Here's how the part is built. I have some questions about the finished solid (model axes, mm). A direction names the side the tool comes from. Give positions to 0.01 mm unless a question says otherwise; leave off trailing zeros. Write each loop counter-clockwise with the first axis right and the second up, starting at its lowest first coordinate (ties: lowest second). Pieces come first, ordered by that corner, then holes. Notation, with made-up numbers: (22.25, -35.75) - (38.25, -35.75) arc R19 cw to (38.25, -0.75) - close; hole circle Ø1 at (67, 33.5). An arc over 180 degrees is marked (long way). One line per item, written item: value. Start each with the question number.
1) On a 3-axis mill with a long thin cutter (end or side, diameter ignored), from which of +Z, -Z, +X, -X, +Y, -Y can I reach the whole of each face in a straight line? I mean faces 1 (the cylindrical face through (20.047, 1.521, -9.306)), 2 (the cylindrical face through (43.04, 1.52, -42.1)). Say none if no direction works.
2) We'd pull the mould along X, two halves only. Please class faces 3 (the flat face through (-1, 1, -42.956)), 4 (the cylindrical face through (0.44, 1.48, 22.88)), 5 (the flat face through (43.941, 1, -17)): +X half, -X half, draft (parallel to the pull), parting line (faces both ways), or undercut.
3) Please list where these lines run through material, in increasing order: L1, parallel to X at y = 1.25, z = 0; L2, parallel to X at y = 2.25, z = 14.5; L3, parallel to Z at x = 0.5, y = 1.6. Write a range as [from, to].
4) Imagine slicing it at A-A on z = 0. Write out the boundary of the cut face in (x, y).
5) Imagine slicing it at B-B on y = 0.65. Count the separate pieces of the cut face and the enclosed holes in it, plus the area to 3 significant figures.
6) I'm going to push flat-ended pins straight in: P1, Ø1, axis at y = 2, z = 10, coming from the -X side; P2, Ø1.5, axis at y = 1.5, z = 17.5, coming from the +X side; P3, Ø1.5, axis at y = 2, z = 19.5, coming from the -X side. Where does each tip first touch, or does it pass through?
from build123d import *

# Parameters (mm, degrees)
SKETCH_2_R      = 1.95
SKETCH_2_R_2    = 1.45
EXTRUDE_3_DEPTH = 3
FILLET_2_R      = 3


with BuildPart() as part:
    # 草图2 → 凸台-拉伸3 (new body)
    with BuildSketch(Plane(origin=(0, 0, 0), x_dir=(1, 0, 0), z_dir=(0, 1, 0))):
        Polygon((-43.941125497, -7.5), (-43.941125497, 7.5), (-43.941125497, 42.955844123), (43.941125497, 42.955844123), (43.941125497, 7.5), (43.941125497, -7.5), (7.5, -7.5), (7.5, -28.5), (-7.5, -28.5), (-7.5, -7.5), align=None)
        with Locations(Location((25.455844123, 24.470562748, 0), (0, 0, 270))):
            Circle(SKETCH_2_R, mode=Mode.SUBTRACT)
        with Locations(Location((33.941125497, 32.955844123, 0), (0, 0, 270))):
            Circle(SKETCH_2_R, mode=Mode.SUBTRACT)
        with Locations(Location((7.5, 0, 0), (0, 0, 270))):
            Circle(SKETCH_2_R, mode=Mode.SUBTRACT)
        with Locations(Location((22.5, 0, 0), (0, 0, 270))):
            Circle(SKETCH_2_R, mode=Mode.SUBTRACT)
        with Locations(Location((-33.941125497, 32.955844123, 0), (0, 0, 90))):
            Circle(SKETCH_2_R, mode=Mode.SUBTRACT)
        with Locations(Location((-25.455844123, 24.470562748, 0), (0, 0, 90))):
            Circle(SKETCH_2_R, mode=Mode.SUBTRACT)
        with Locations(Location((-22.5, 0, 0), (0, 0, 90))):
            Circle(SKETCH_2_R, mode=Mode.SUBTRACT)
        with Locations(Location((-7.5, 0, 0), (0, 0, 90))):
            Circle(SKETCH_2_R, mode=Mode.SUBTRACT)
        with Locations(Location((0, -14.5, 0), (0, 0, 270))):
            Circle(SKETCH_2_R_2, mode=Mode.SUBTRACT)
        with Locations(Location((0, -21.5, 0), (0, 0, 270))):
            Circle(SKETCH_2_R_2, mode=Mode.SUBTRACT)
        Polygon((38.941125497, 30.884776311), (15.556349186, 7.5), (38.941125497, 7.5), align=None, mode=Mode.SUBTRACT)
        Polygon((-15.556349186, 7.5), (-38.941125497, 7.5), (-38.941125497, 30.884776311), align=None, mode=Mode.SUBTRACT)
        Polygon((24.798989873, 37.955844123), (0, 13.156854249), (-24.798989873, 37.955844123), align=None, mode=Mode.SUBTRACT)
    extrude(amount=EXTRUDE_3_DEPTH)

    # 圆角2
    fillet_2_edges = [part.edges().sort_by_distance(p)[0] for p in [
        (43.941125497, 1.5, 7.5),
        (7.5, 1.5, 7.5),
        (7.5, 1.5, 28.5),
        (-7.5, 1.5, 28.5),
        (-7.5, 1.5, 7.5),
        (-43.941125497, 1.5, 7.5),
        (-43.941125497, 1.5, -42.955844123),
        (43.941125497, 1.5, -42.955844123),
        (38.941125497, 1.5, -7.5),
        (38.941125497, 1.5, -30.884776311),
        (15.556349186, 1.5, -7.5),
        (-15.556349186, 1.5, -7.5),
        (-38.941125497, 1.5, -30.884776311),
        (-38.941125497, 1.5, -7.5),
        (24.798989873, 1.5, -37.955844123),
        (-24.798989873, 1.5, -37.955844123),
        (0, 1.5, -13.156854249),
    ]]
    fillet(fillet_2_edges, radius=FILLET_2_R)


solid = part.part
Numbers:
1. face 1: +Y, -Y
1. face 2: -Z, +X, +Y, -Y
2. face 3: draft
2. face 4: undercut
2. face 5: +X half
3. L1: [-43.94, -24.45], [-20.55, -9.45], [-5.55, 5.55], [9.45, 20.55], [24.45, 43.94]
3. L2: [-7.5, -1.45], [1.45, 7.5]
3. L3: [-42.96, -37.96], [-14.44, 13.14], [15.86, 20.14], [22.86, 28.5]
4. outline: (-43.94, 0) - (-24.45, 0) - (-24.45, 3) - (-43.94, 3) - close; (-20.55, 0) - (-9.45, 0) - (-9.45, 3) - (-20.55, 3) - close; (-5.55, 0) - (5.55, 0) - (5.55, 3) - (-5.55, 3) - close; (9.45, 0) - (20.55, 0) - (20.55, 3) - (9.45, 3) - close; (24.45, 0) - (43.94, 0) - (43.94, 3) - (24.45, 3) - close
5. separate pieces: 1
5. enclosed holes: 13
5. area: 3,540 mm^2
6. P1: x = -7.67
6. P2: x = 7.5
6. P3: x = -7.5
